The listing builds one solid part. Answer for the finished solid, in the listing's coordinates (mm). Round coordinates to 2 decimals unless told otherwise and drop trailing zeros. Write each loop counter-clockwise with the first axis right and the second up, starting at its lowest first coordinate (ties: lowest second). Pieces come first, ordered by that corner, then holes.
from build123d import *

# Parameters (mm, degrees)
F1_DEPTH = 15
F2_R     = 5.08
F4_D     = 6.35


with BuildPart() as f1:
    # F0 (on Right) → F1 (new body)
    with BuildSketch(Plane.YZ):
        Polygon((10.627066, 24.493142), (-21.372934, 24.493142), (-21.372934, -4.169433), (3.627066, -4.169433), align=None)
    extrude(amount=F1_DEPTH)

    # F2
    f2_edges = [f1.edges().sort_by_distance(p)[0] for p in [
        (15, -21.372934, 10.161854),
        (15, -5.372934, 24.493142),
        (7.5, -21.372934, 24.493142),
    ]]
    fillet(f2_edges, radius=F2_R)

    # F4 (through all)
    with Locations(Plane.YZ.offset(15)):
        with Locations((-7.430566, 12.076859)):
            Hole(F4_D / 2)


solid = f1.part
1. Straight lines are drawn through the part: line 1 along Z through (x, y) = (4.5, -5.5); line 2 along Z through (x, y) = (9, -8.5); line 3 along Y through (x, z) = (12.5, 22.75). For each, find the intervals that lie inside material, in ascending order.
Geometry says:
line 1: z = -4.17 to 9.56, 14.6 to 24.49
line 2: z = -4.17 to 9.09, 15.07 to 24.49
line 3: y = -19.12 to 10.2
2. Section A-A on y = -5 is taken. Determine the outline of the cut face in (x, z), plus the area to 3 significant figures.
Geometry says:
outline: (0, -4.17) - (15, -4.17) - (15, 10.03) - (0, 10.03) - close; (0, 14.12) - (15, 14.12) - (15, 19.41) arc R5.08 ccw to (9.92, 24.49) - (0, 24.49) - close
area: 363 mm2
3. Given pin 1 (4 mm diameter, centred on x = 2, z = 12.5, fed in from +Y); pin 2 (8.5 mm diameter, centred on y = -7.43, z = 12.08, fed in from +X); pin 3 (2 mm diameter, centred on x = 13, z = 7, fed in from +Y); pin 4 (4 mm diameter, centred on x = 13, y = -16, fed in from +Z), each flat-ended and moving along its own axis, determine where each tip first touches the part or whether it passes through.
Geometry says:
pin 1: stops at y = 8.19
pin 2: stops at x = 15
pin 3: stops at y = 6.6
pin 4: stops at z = 24.38
4. Section C-C on x = 12.5 is taken. Determine the outline of the cut face in (y, z) (3 decimals).
Geometry says:
outline: (-20.669, -4.169) - (3.627, -4.169) - (10.455, 23.789) - (-16.293, 23.789) arc R4.376 ccw to (-20.669, 19.413) - close; hole circle Ø6.35 at (-7.431, 12.077)
5. Section D-D on y = 6 is taken. Determine the outline of the cut face in (x, z).
Geometry says:
outline: (0, 5.55) - (15, 5.55) - (15, 19.41) arc R5.08 ccw to (9.92, 24.49) - (0, 24.49) - close
6. Section B-B on z = 9.75 is taken. Determine the outline of the cut face in (x, y), plus the area to 3 significant figures.
Geometry says:
outline: (0, -21.37) - (9.92, -21.37) arc R5.08 ccw to (15, -16.29) - (15, -9.59) - (0, -9.59) - close; (0, -5.27) - (15, -5.27) - (15, 7.03) - (0, 7.03) - close
area: 356 mm2
